from build123d import *

# Parameters (mm, degrees)
SCHIZZO1_W                   = 394.303075113
SCHIZZO1_H                   = 40
SCHIZZO1_R                   = 6
ESTRUSIONE_ESTRUSIONE1_DEPTH = 5


with BuildPart() as part:
    # Schizzo1 → Estrusione-Estrusione1 (new, symmetric)
    with BuildSketch(Plane.XY):
        with Locations((177.151537557, 119.723097721)):
            Rectangle(SCHIZZO1_W, SCHIZZO1_H)
        with Locations((0, 128.056431054)):
            Circle(SCHIZZO1_R, mode=Mode.SUBTRACT)
        with Locations(Location((354.303075113, 128.056431054, 0), (0, 0, 180))):
            Circle(SCHIZZO1_R, mode=Mode.SUBTRACT)
    extrude(amount=ESTRUSIONE_ESTRUSIONE1_DEPTH, both=True)


solid = part.part
For this review, take the finished solid that the model builds, in its own axes (mm). Round coordinates to 2 decimals unless told otherwise and drop trailing zeros. Write each loop counter-clockwise with the first axis right and the second up, starting at its lowest first coordinate (ties: lowest second). Pieces come first, ordered by that corner, then holes. Notation, with made-up numbers: (52, 55.25) -> (92, 55.25) arc R12 cw to (92, 69.25) -> close; hole circle Ø6 at (13, 82.5). An arc over 180 degrees is marked (long way). Put each result on its own line as item: value.
Q1. To check wall thickness, follow L1, parallel to X at y = 129, z = 1; L2, parallel to X at y = 128, z = 3.75; L3, parallel to Y at x = 0, z = -0.5. State the ranges of each line that lie inside material, in increasing order. Write a range as [from, to].
Determined:
L1: x = [-20, -5.93], [5.93, 348.38], [360.23, 374.3]
L2: x = [-20, -6], [6, 348.3], [360.3, 374.3]
L3: y = [99.72, 122.06], [134.06, 139.72]
Q2. Clearance check with a flat-ended pin moving along its axis: pin 1 Ø9.5 at (x, y) = (0, 128.06) entering from -Z. State where the tip first meets the part, or that it passes through.
Determined:
pin 1: passes through
Q3. Consider section A-A on x = 0. State the section outline as (y, z) points.
Determined:
outline: (99.72, -5) -> (122.06, -5) -> (122.06, 5) -> (99.72, 5) -> close; (134.06, -5) -> (139.72, -5) -> (139.72, 5) -> (134.06, 5) -> close
Q4. The part is to be moulded in two halves that separate along Y. For faces 1 (the cylindrical face through (-1.3, 122.2, -0.1)), 2 (the flat face through (174, 120, 5)), 3 (the flat face through (174, 99.723, 0)), say which applies: released by +Y, released by -Y, zero draft, split by the parting line, or undercut.
Determined:
face 1: undercut
face 2: zero draft
face 3: released by -Y
